Work out the finished part from the listing and answer in its coordinate system (mm). Face numbers are marked on the shaded views. A direction names the side the tool comes from. Round coordinates to 2 decimals unless told otherwise and drop trailing zeros. Write each loop counter-clockwise with the first axis right and the second up, starting at its lowest first coordinate (ties: lowest second). Pieces come first, ordered by that corner, then holes. Notation, with made-up numbers: (66, 34) -> (82, 34) arc R19 ccw to (82, 62) -> close; hole circle Ø4 at (48.5, 11.25). An arc over 180 degrees is marked (long way). One line per question, with ' | ' between items. Start each with the question number.
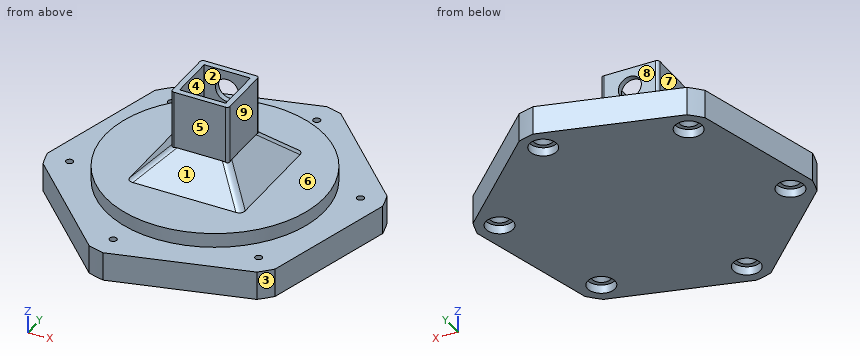
```python
from build123d import *

# Parameters (mm, degrees)
SKETCH_1_R          = 53.5
EXTRUDE_1_DEPTH     = 10
SKETCH_2_R          = 38
EXTRUDE_2_DEPTH     = 5
SKETCH_3_W          = 20
SKETCH_3_H          = 20
SKETCH_3_W_2        = 16
SKETCH_3_H_2        = 16
EXTRUDE_3_DEPTH     = 30
SKETCH_4_R          = 3
CUT_EXTRUDE_1_DEPTH = 19
CHAMFER_1_SIZE      = 10
FILLET_1_R          = 3
FILLET_2_R          = 1
SKETCH_6_W          = 16
SKETCH_6_H          = 16
CUT_EXTRUDE_2_DEPTH = 35
CUT_EXTRUDE_3_DEPTH = 16
SKETCH_8_R          = 1.25
CUT_EXTRUDE_4_DEPTH = 20
SKETCH_9_R          = 4.75
CUT_EXTRUDE_5_DEPTH = 3
SKETCH_10_R         = 4
CUT_EXTRUDE_6_DEPTH = 5


with BuildPart() as part:
    # Эскиз1 → Бобышка-Вытянуть1 (new body)
    with BuildSketch(Plane.XY):
        Circle(SKETCH_1_R)
    extrude(amount=-EXTRUDE_1_DEPTH)

    # Эскиз2 → Бобышка-Вытянуть2 (add)
    with BuildSketch(Plane.XY):
        Circle(SKETCH_2_R)
    extrude(amount=EXTRUDE_2_DEPTH)

    # Эскиз3 → Бобышка-Вытянуть3 (add)
    with BuildSketch(Plane.XY.offset(5)):
        Rectangle(SKETCH_3_W, SKETCH_3_H)
        Rectangle(SKETCH_3_W_2, SKETCH_3_H_2, mode=Mode.SUBTRACT)
    extrude(amount=EXTRUDE_3_DEPTH)

    # Эскиз4 → Вырез-Вытянуть1 (cut)
    with BuildSketch(Plane.ZY.offset(10)):
        with Locations(Location((20, 0, 0), (0, 0, 270))):
            Circle(SKETCH_4_R)
    extrude(amount=-CUT_EXTRUDE_1_DEPTH, mode=Mode.SUBTRACT)

    # Фаска1
    chamfer_1_edges = [part.edges().sort_by_distance(p)[0] for p in [
        (10, 0, 5),
        (0, 10, 5),
        (-10, 0, 5),
        (0, -10, 5),
    ]]
    chamfer(chamfer_1_edges, length=CHAMFER_1_SIZE)

    # Скругление1
    fillet_1_edges = [part.edges().sort_by_distance(p)[0] for p in [
        (15, -15, 10),
        (-15, -15, 10),
        (15, 15, 10),
        (-15, 15, 10),
    ]]
    fillet(fillet_1_edges, radius=FILLET_1_R)

    # Fillet 2
    fillet_2_edges = [part.edges().sort_by_distance(p)[0] for p in [
        (-10, -10, 24.715796964),
        (-10, 10, 24.715796964),
        (10, 10, 24.715796964),
        (10, -10, 24.715796964),
    ]]
    fillet(fillet_2_edges, radius=FILLET_2_R)

    # Эскиз6 → Вырез-Вытянуть2 (cut)
    with BuildSketch(Plane.XY.offset(35)):
        Rectangle(SKETCH_6_W, SKETCH_6_H)
    extrude(amount=-CUT_EXTRUDE_2_DEPTH, mode=Mode.SUBTRACT)

    # Эскиз7 → Вырез-Вытянуть3 (cut)
    with BuildSketch(Plane.XY):
        with BuildLine():
            Line((-50.83668087, -16.669789385), (-16.669789385, -50.83668087))
            ThreePointArc((-16.669789385, -50.83668087), (-37.830212793, -37.830212793), (-50.83668087, -16.669789385))
        make_face()
        with BuildLine():
            Line((-39.854801518, 35.690962385), (-52.36075177, -10.981879352))
            ThreePointArc((-52.36075177, -10.981879352), (-51.677031706, 13.846818913), (-39.854801518, 35.690962385))
        make_face()
        with BuildLine():
            Line((10.981879352, 52.36075177), (-35.690962385, 39.854801518))
            ThreePointArc((-35.690962385, 39.854801518), (-13.846818913, 51.677031706), (10.981879352, 52.36075177))
        make_face()
        with BuildLine():
            Line((50.83668087, 16.669789385), (16.669789385, 50.83668087))
            ThreePointArc((16.669789385, 50.83668087), (37.830212793, 37.830212793), (50.83668087, 16.669789385))
        make_face()
        with BuildLine():
            Line((39.854801518, -35.690962385), (52.36075177, 10.981879352))
            ThreePointArc((52.36075177, 10.981879352), (51.677031706, -13.846818913), (39.854801518, -35.690962385))
        make_face()
        with BuildLine():
            Line((-10.981879352, -52.36075177), (35.690962385, -39.854801518))
            ThreePointArc((35.690962385, -39.854801518), (13.846818913, -51.677031706), (-10.981879352, -52.36075177))
        make_face()
    extrude(amount=-CUT_EXTRUDE_3_DEPTH, mode=Mode.SUBTRACT)

    # Эскиз8 → Вырез-Вытянуть4 (cut)
    with BuildSketch(Plane(origin=(0, 0, -10), x_dir=(-1, 0, 0), z_dir=(0, 0, -1))):
        with Locations((32.350135239, 32.350135239)):
            Circle(SKETCH_8_R)
        with Locations((44.191106553, -11.840971313)):
            Circle(SKETCH_8_R)
        with Locations((11.840971313, -44.191106553)):
            Circle(SKETCH_8_R)
        with Locations((-32.350135239, -32.350135239)):
            Circle(SKETCH_8_R)
        with Locations((-44.191106553, 11.840971313)):
            Circle(SKETCH_8_R)
        with Locations((-11.840971313, 44.191106553)):
            Circle(SKETCH_8_R)
    extrude(amount=-CUT_EXTRUDE_4_DEPTH, mode=Mode.SUBTRACT)

    # Эскиз9 → Вырез-Вытянуть5 (cut)
    with BuildSketch(Plane(origin=(0, 0, -10), x_dir=(-1, 0, 0), z_dir=(0, 0, -1))):
        with Locations((-11.840971313, 44.191106553)):
            Circle(SKETCH_9_R)
        with Locations((-44.191106553, 11.840971313)):
            Circle(SKETCH_9_R)
        with Locations((-32.350135239, -32.350135239)):
            Circle(SKETCH_9_R)
        with Locations((11.840971313, -44.191106553)):
            Circle(SKETCH_9_R)
        with Locations((44.191106553, -11.840971313)):
            Circle(SKETCH_9_R)
        with Locations((32.350135239, 32.350135239)):
            Circle(SKETCH_9_R)
    extrude(amount=-CUT_EXTRUDE_5_DEPTH, mode=Mode.SUBTRACT)

    # Fillet 2 2: read off the stored shape, not the designer's step
    # Fillet 2 2 outline → Fillet 2 2 (revolve, cut)
    with BuildSketch(Plane(origin=(-11.840971313, -44.191106553, 0), x_dir=(1, 0, 0), z_dir=(0, -1, 0))):
        Polygon((3.25, -7), (1.25, -5), (1.25, -7), align=None)
    revolve(axis=Axis((-11.840971313, -44.191106553, 0), (0, 0, 1)), mode=Mode.SUBTRACT)

    # Фаска3: read off the stored shape, not the designer's step
    # Фаска3 outline → Фаска3 (revolve, cut)
    with BuildSketch(Plane(origin=(32.350135239, -32.350135239, 0), x_dir=(1, 0, 0), z_dir=(0, -1, 0))):
        Polygon((3.25, -7), (1.25, -5), (1.25, -7), align=None)
    revolve(axis=Axis((32.350135239, -32.350135239, 0), (0, 0, 1)), mode=Mode.SUBTRACT)

    # Фаска4: read off the stored shape, not the designer's step
    # Фаска4 outline → Фаска4 (revolve, cut)
    with BuildSketch(Plane(origin=(44.191106553, 11.840971313, 0), x_dir=(1, 0, 0), z_dir=(0, -1, 0))):
        Polygon((3.25, -7), (1.25, -5), (1.25, -7), align=None)
    revolve(axis=Axis((44.191106553, 11.840971313, 0), (0, 0, 1)), mode=Mode.SUBTRACT)

    # Фаска5: read off the stored shape, not the designer's step
    # Фаска5 outline → Фаска5 (revolve, cut)
    with BuildSketch(Plane(origin=(11.840971313, 44.191106553, 0), x_dir=(1, 0, 0), z_dir=(0, -1, 0))):
        Polygon((3.25, -7), (1.25, -5), (1.25, -7), align=None)
    revolve(axis=Axis((11.840971313, 44.191106553, 0), (0, 0, 1)), mode=Mode.SUBTRACT)

    # Фаска6: read off the stored shape, not the designer's step
    # Фаска6 outline → Фаска6 (revolve, cut)
    with BuildSketch(Plane(origin=(-32.350135239, 32.350135239, 0), x_dir=(1, 0, 0), z_dir=(0, -1, 0))):
        Polygon((3.25, -7), (1.25, -5), (1.25, -7), align=None)
    revolve(axis=Axis((-32.350135239, 32.350135239, 0), (0, 0, 1)), mode=Mode.SUBTRACT)

    # Фаска7: read off the stored shape, not the designer's step
    # Фаска7 outline → Фаска7 (revolve, cut)
    with BuildSketch(Plane(origin=(-44.191106553, -11.840971313, 0), x_dir=(1, 0, 0), z_dir=(0, -1, 0))):
        Polygon((3.25, -7), (1.25, -5), (1.25, -7), align=None)
    revolve(axis=Axis((-44.191106553, -11.840971313, 0), (0, 0, 1)), mode=Mode.SUBTRACT)

    # Эскиз10 → Вырез-Вытянуть6 (cut)
    with BuildSketch(Plane(origin=(0, 10, 0), x_dir=(1, 0, 0), z_dir=(0, 1, 0))):
        with Locations(Location((-0.060660172, -28, 0), (0, 0, 270))):
            Circle(SKETCH_10_R)
    extrude(amount=-CUT_EXTRUDE_6_DEPTH, mode=Mode.SUBTRACT)


solid = part.part
```
(1) A cutting plane is placed at C-C, the plane x = 23. Determine the outline of the cut face in (y, z), then the cut area to 3 significant figures.
(2) A cutting plane is placed at B-B, the plane y = 0. Determine the outline of the cut face in (x, z), then the cut area to 3 significant figures.
(3) Given pin 1 Ø12.5 at (x, y) = (-11.84, -44.19) entering from -Z; pin 2 Ø9 at (y, z) = (-4.5, 26.5) entering from -X; pin 3 Ø4 at (x, z) = (29.5, 5) entering from +Y (3 decimals); pin 4 Ø3 at (x, z) = (7.5, 11.5) entering from +Y, each flat-ended and moving along its own axis, determine where each tip first touches the part or whether it passes through.
(4) A cutting plane is placed at A-A, the plane z = 20. Determine the outline of the cut face in (x, y), then the cut area to 3 significant figures.
(5) Consider L1, parallel to Z at x = -9.15, y = 0; L2, parallel to Z at x = 11, y = 32.5; L3, parallel to Z at x = 43, y = 4.5. Determine where each line is inside the solid, lowest interval first.
(6) For the marked faces 5, 6, 7, 8 and 9, determine the directions among +Z, -Z, +X, -X, +Y, -Y from which every point of the face is accessible in a straight line to the end or side of a thin tool.
(7) A cutting plane is placed at D-D, the plane z = 28. Determine the outline of the cut face in (x, y), then the cut area to 3 significant figures.
(8) The mould has two halves that part along X. Classify the marked faces 1, 2, 3 and 4: +X half, -X half, draft (parallel to the pull), parting line (faces both ways), or undercut.
Returned:
1) outline: (-43.26, -10) -> (44.51, -10) -> (44.51, 0) -> (30.25, 0) -> (30.25, 5) -> (-30.25, 5) -> (-30.25, 0) -> (-43.26, 0) -> close | area: 1,180 mm2
2) outline: (-49.42, -10) -> (49.42, -10) -> (49.42, 0) -> (38, 0) -> (38, 5) -> (20, 5) -> (10, 15) -> (10, 35) -> (8, 35) -> (8, 23) -> (9, 23) -> (9, 17) -> (8, 17) -> (8, 0) -> (-8, 0) -> (-8, 17) -> (-10, 17) -> (-10, 15) -> (-20, 5) -> (-38, 5) -> (-38, 0) -> (-49.42, 0) -> close; (-10, 23) -> (-8, 23) -> (-8, 35) -> (-10, 35) -> close | area: 1,490 mm2
3) pin 1: z = -10 | pin 2: x = -10 | pin 3: y = 26.225 | pin 4: y = 15
4) outline: (-10, -9) arc R1 ccw to (-9, -10) -> (9, -10) arc R1 ccw to (10, -9) -> (10, 9) arc R1 ccw to (9, 10) -> (-9, 10) arc R1 ccw to (-10, 9) -> (-10, 3) -> (-8, 3) -> (-8, 8) -> (8, 8) -> (8, 3) -> (9, 3) -> (9, -3) -> (8, -3) -> (8, -8) -> (-8, -8) -> (-8, -3) -> (-10, -3) -> close | area: 125 mm2
5) L1: -10 to 17, 23 to 35 | L2: -10 to 5 | L3: -10 to 0
6) face 5: +Z, +X, -X, -Y | face 6: +Z | face 7: +Z, -X, +Y, -Y | face 8: +Z, +X, -X, +Y | face 9: +Z, +X, +Y, -Y
7) outline: (-10, -9) arc R1 ccw to (-9, -10) -> (9, -10) arc R1 ccw to (10, -9) -> (10, 9) arc R1 ccw to (9, 10) -> (3.94, 10) -> (3.94, 8) -> (8, 8) -> (8, -8) -> (-8, -8) -> (-8, 8) -> (-4.06, 8) -> (-4.06, 10) -> (-9, 10) arc R1 ccw to (-10, 9) -> close | area: 127 mm2
8) face 1: draft | face 2: undercut | face 3: +X half | face 4: undercut
